Source: CAD feature listing. Evaluate the final solid. Frame: model axes, mm. Round coordinates to 2 decimals unless told otherwise and drop trailing zeros. Loops run counter-clockwise (first coordinate to the right, second up) from the corner with the lowest first, then second, coordinate; pieces in that order, holes last.
Item 1: Section query A-A on y = -1.05. Give the number of separate pieces and of enclosed holes in the cut face, then the cut area to 3 significant figures.
Item 2: First-contact query: P1, Ø0.7, axis at x = -7, y = -1, coming from the +Z side; P2, Ø1.1, axis at y = -2, z = 7.5, coming from the -X side; P3, Ø6, axis at x = 6.05, z = 111.24, coming from the +Y side. Flat tips, straight axial feed; report the tip coordinate or a pass-through.
Item 3: Section query C-C on z = 49.5. Return loops of the section in (x, y), then the cut area to 3 significant figures.
Item 4: Ray query, L1, parallel to Z at x = 4, y = -0.6; L2, parallel to Z at x = -28, y = -0.2; L3, parallel to Z at x = -6.5, y = -0.55. Return the intervals inside material, ascending.
Item 5: Section query B-B on x = -25. Return loops of the section in (y, z), then the cut area to 3 significant figures.
```python
from build123d import *

# Parameters (mm, degrees)
F0_R     = 5.08
F0_R_2   = 5.715
F1_DEPTH = 3.048


# Not quite as in the source:
# - a feature of the source that left no trace in its solid (it failed there, or was rolled back) is left out


with BuildPart() as f1:
    # F0 (on Front) → F1 (new body)
    with BuildSketch(Plane.XZ):
        with BuildLine():
            ThreePointArc((0, 57.785), (-5.715, 63.5), (0, 69.215))
            Line((0, 69.215), (0, 126.4542473564))
            ThreePointArc((0, 126.4542473564), (-6.6367069731, 129.1469896364), (-9.5209852919, 135.7027259805))
            Line((-9.5209852919, 135.7027259805), (-15.8126809955, 64.9052561096))
            Line((-15.8126809955, 64.9052561096), (-10.0230526485, 16.8384262865))
            ThreePointArc((-10.0230526485, 16.8384262865), (-11.9679184287, 10.6128911922), (-17.9162015492, 7.9375))
            Line((-17.9162015492, 7.9375), (-44.45, 7.9375))
            ThreePointArc((-44.45, 7.9375), (-38.8373399243, 5.6126600757), (-36.5125, 0))
            Line((-36.5125, 0), (-7.9375, 0))
            ThreePointArc((-7.9375, 0), (-5.6126600757, 5.6126600757), (0, 7.9375))
            Line((0, 7.9375), (0, 57.785))
        make_face()
        with BuildLine():
            Line((0, 126.4542473564), (0, 69.215))
            ThreePointArc((0, 69.215), (4.0411152545, 67.5411152545), (5.715, 63.5))
            ThreePointArc((5.715, 63.5), (4.0411152545, 59.4588847455), (0, 57.785))
            Line((0, 57.785), (0, 7.9375))
            ThreePointArc((0, 7.9375), (5.6126600757, 5.6126600757), (7.9375, 0))
            Line((7.9375, 0), (15.8132155809, 64.8992276415))
            Line((15.8132155809, 64.8992276415), (9.5249892223, 135.9649185116))
            ThreePointArc((9.5249892223, 135.9649185116), (6.7301241724, 129.2389911578), (0, 126.4542473564))
        make_face()
        with Locations((6.0517773964, 111.243724823)):
            Circle(F0_R, mode=Mode.SUBTRACT)
        with BuildLine():
            ThreePointArc((-9.5209852919, 135.7027259805), (-6.6367069731, 129.1469896364), (0, 126.4542473564))
            ThreePointArc((0, 126.4542473564), (6.7301241724, 129.2389911578), (9.5249892223, 135.9649185116))
            ThreePointArc((9.5249892223, 135.9649185116), (9.5249973056, 135.972082932), (9.525, 135.9792473564))
            ThreePointArc((9.525, 135.9792473564), (-0.1382752592, 145.5032436265), (-9.5209852919, 135.7027259805))
        make_face()
        with BuildLine():
            ThreePointArc((5.715, 135.9792473564), (4.0411152545, 131.9381321019), (0, 130.2642473564))
            ThreePointArc((0, 130.2642473564), (-4.0411152545, 140.0203626109), (5.715, 135.9792473564))
        make_face(mode=Mode.SUBTRACT)
        with BuildLine():
            ThreePointArc((7.9375, 0), (5.6126600757, 5.6126600757), (0, 7.9375))
            Line((0, 7.9375), (0, 5.715))
            ThreePointArc((0, 5.715), (4.0411152545, 4.0411152545), (5.715, 0))
            ThreePointArc((5.715, 0), (0, -5.715), (-5.715, 0))
            Line((-5.715, 0), (-7.9375, 0))
            ThreePointArc((-7.9375, 0), (-5.6126600757, -5.6126600757), (0, -7.9375))
            ThreePointArc((0, -7.9375), (5.6126600757, -5.6126600757), (7.9375, 0))
        make_face()
        with BuildLine():
            ThreePointArc((0, -7.9375), (-5.6126600757, -5.6126600757), (-7.9375, 0))
            Line((-7.9375, 0), (-36.5125, 0))
            ThreePointArc((-36.5125, 0), (-38.8373399243, -5.6126600757), (-44.45, -7.9375))
            Line((-44.45, -7.9375), (0, -7.9375))
        make_face()
        with BuildLine():
            ThreePointArc((-44.45, -7.9375), (-38.8373399243, -5.6126600757), (-36.5125, 0))
            ThreePointArc((-36.5125, 0), (-38.8373399243, 5.6126600757), (-44.45, 7.9375))
            ThreePointArc((-44.45, 7.9375), (-52.3875, 0), (-44.45, -7.9375))
        make_face()
        with Locations((-44.45, 0)):
            Circle(F0_R_2, mode=Mode.SUBTRACT)
    extrude(amount=F1_DEPTH)


solid = f1.part
```
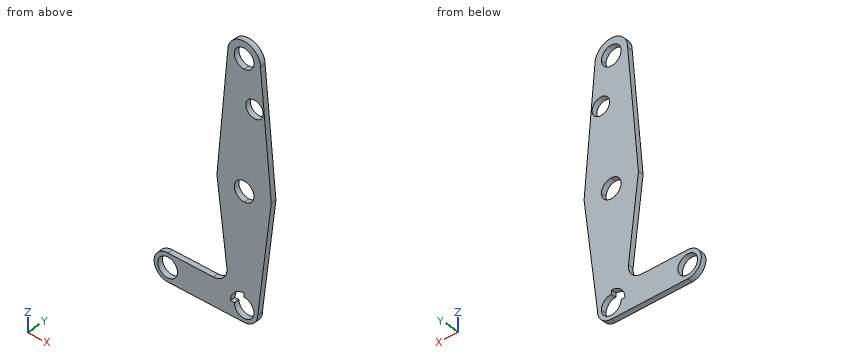
Data:
1. separate pieces: 1
1. enclosed holes: 5
1. area: 3,780 mm2
2. P1: stops at z = 142.8
2. P2: stops at x = -48.28
2. P3: passes through
3. outline: (-13.96, -3.05) - (13.94, -3.05) - (13.94, 0) - (-13.96, 0) - close
3. area: 85.0 mm2
4. L1: z = -6.86 to -4.08, 4.08 to 59.42, 67.58 to 106.6, 115.89 to 131.9, 140.06 to 144.62
4. L2: z = -7.94 to 7.94
4. L3: z = -7.94 to 0, 4.56 to 142.94
5. outline: (-3.05, -7.94) - (0, -7.94) - (0, 7.94) - (-3.05, 7.94) - close
5. area: 48.4 mm2
